Verification items for the finished model (mm, model axes). A direction names the side the tool comes from. Give positions to 0.01 mm unless a question says otherwise; leave off trailing zeros. Write each loop counter-clockwise with the first axis right and the second up, starting at its lowest first coordinate (ties: lowest second). Pieces come first, ordered by that corner, then holes. Notation, with made-up numbers: (41.5, 71.5) - (49.5, 71.5) arc R27 ccw to (49.5, 109.5) - close; hole circle Ø10 at (49, -29.5). An arc over 180 degrees is marked (long way). Answer as a JSON object with one key per item and string values. Group by question number.
Item 1: Sectioned sample at B-B, the plane x = 2.5. Record the boundary of the cut face in (y, z).
Item 2: Sectioned sample at C-C, the plane z = 1. Record the boundary of the cut face in (x, y), and give its area (3 significant figures).
Item 3: Draft check along Z on faces 1 (the face through (-3.16, 2.33, 0.4)), 2 (the face through (0.49, -4.88, 1.08)), 3 (the face through (0, -2, 0)). Enter one of: +Z half, -Z half, draft (parallel to the pull), parting line (faces both ways), or undercut.
Item 4: Scan lines: line 1 along Y through (x, z) = (2, 0); line 2 along Z through (x, y) = (-3, 0.75); line 3 along X through (y, z) = (2.25, 2.75). Record each from-to range of solid material in increasing order. Write a range as [from, to].
Item 5: Go/stop test with flat-tipped pins: pin 1 (4 mm diameter, centred on x = 0, z = -3, fed in from +Y); pin 2 (2.5 mm diameter, centred on y = 0, z = 0, fed in from +X); pin 3 (2 mm diameter, centred on x = -4, y = 2, fed in from +Z); pin 4 (4 mm diameter, centred on x = -4, z = -1, fed in from +Y). Record where each tip stops, or that it passes through.
Item 6: Sectioned sample at A-A, the plane z = 0. Record the boundary of the cut face in (x, y).
Item 7: Tool access check on faces 4 (the face through (-0.823, -0.67, 1.617)), 5 (the face through (3.465, -0.67, -1.617)), 6 (the face through (-4, 2.493, 1)). Record the directions out of +Z, -Z, +X, -X, +Y, -Y that give a thin tool (end or side, any length) a straight path to the whole face; none if there is none.
Item 8: Sectioned sample at D-D, the plane y = -3.5. Record the boundary of the cut face in (x, z), and give its area (3 significant figures).
```python
from build123d import *

# Parameters (mm, degrees)
SKETCH1_R           = 5
BOSS_EXTRUDE1_DEPTH = 1
SKETCH2_R           = 1.75
SKETCH2_R_2         = 0.75
BOSS_EXTRUDE2_DEPTH = 5
SKETCH4_R           = 0.75
CUT_EXTRUDE1_DEPTH  = 10
SKETCH5_R           = 1.75
SKETCH5_R_2         = 0.75


with BuildPart() as part:
    # Sketch1 → Boss-Extrude1 (new body)
    with BuildSketch(Plane(origin=(0, 0, 0), x_dir=(0, 0, -1), z_dir=(1, 0, 0))):
        Circle(SKETCH1_R)
    extrude(amount=BOSS_EXTRUDE1_DEPTH)

    # Sketch2 → Boss-Extrude2 (add)
    with BuildSketch(Plane(origin=(1, 0, 0), x_dir=(0, 0, -1), z_dir=(1, 0, 0))):
        Circle(SKETCH2_R)
        Circle(SKETCH2_R_2, mode=Mode.SUBTRACT)
    extrude(amount=BOSS_EXTRUDE2_DEPTH)

    # Sketch4 → Cut-Extrude1 (cut)
    with BuildSketch(Plane.ZY):
        Circle(SKETCH4_R)
    extrude(amount=-CUT_EXTRUDE1_DEPTH, mode=Mode.SUBTRACT)

    # Sweep5: sweep along a path in Sketch6
    with BuildLine(Plane.XY) as sweep5_path:
        Line((0, 1.75), (-1.62315873, 1.75))
        ThreePointArc((-1.62315873, 1.75), (-1.921825037, 1.873711635), (-2.045536672, 2.172377942))
        Line((-2.045536672, 2.172377942), (-2.045536672, 2.4927445))
    # Sketch5 → Sweep5 (sweep)
    with BuildSketch(Plane.ZY):
        Circle(SKETCH5_R)
        Circle(SKETCH5_R_2, mode=Mode.SUBTRACT)
    sweep(path=sweep5_path.line)


solid = part.part
```
Geometry check:
{
 "1": {"outline": "circle Ø3.5 at (0, 0); hole circle Ø1.5 at (0, 0)"},
 "2": {"outline": "(-5.23, 2.17) arc R3.61 ccw to (-1.62, -1.44) - (0, -1.44) - (0, -4.9) - (1, -4.9) - (1, -1.44) - (6, -1.44) - (6, 1.44) - (1, 1.44) - (1, 4.9) - (0, 4.9) - (0, 1.44) - (-1.62, 1.44) arc R0.74 cw to (-2.36, 2.17) - (-2.36, 2.49) - (-5.23, 2.49) - close", "area": "39.5 mm^2"},
 "3": {"face 1": "undercut", "face 2": "parting line", "face 3": "draft"},
 "4": {"line 1": "[-1.75, -0.75], [0.75, 1.75]", "line 2": "[-1.74, -0.72], [0.72, 1.74]", "line 3": "[0, 1]"},
 "5": {"pin 1": "y = 4.9", "pin 2": "x = 6", "pin 3": "z = 1.75", "pin 4": "y = 2.49"},
 "6": {"outline": "(-5.55, 2.17) arc R3.92 ccw to (-1.62, -1.75) - (0, -1.75) - (0, -5) - (1, -5) - (1, -1.75) - (6, -1.75) - (6, -0.75) - (-1.62, -0.75) arc R2.92 cw to (-4.55, 2.17) - (-4.55, 2.49) - (-5.55, 2.49) - close; (-3.05, 2.17) arc R1.42 ccw to (-1.62, 0.75) - (6, 0.75) - (6, 1.75) - (1, 1.75) - (1, 5) - (0, 5) - (0, 1.75) - (-1.62, 1.75) arc R0.42 cw to (-2.05, 2.17) - (-2.05, 2.49) - (-3.05, 2.49) - close"},
 "7": {"face 4": "none", "face 5": "+X", "face 6": "+Z, -Z, -X, +Y"},
 "8": {"outline": "(0, -3.57) - (1, -3.57) - (1, 3.57) - (0, 3.57) - close", "area": "7.14 mm^2"}
}
